from build123d import *

# Parameters (mm, degrees)
SKETCH1_W                                       = 295
SKETCH1_H                                       = 60
BOSS_EXTRUDE1_DEPTH                             = 3.175
FILLET1_R                                       = 10
F_3_0MM_DOWEL_HOLE1_D                           = 3
SKETCH6_R                                       = 12.5
CUT_EXTRUDE1_DEPTH                              = 242.888570679
F_6_0MM_DOWEL_HOLE1_D                           = 6
CSK_FOR_M3_FLAT_HEAD_MACHINE_SCREW1_D           = 3.4
CSK_FOR_M3_FLAT_HEAD_MACHINE_SCREW1_CSINK_D     = 6.3
CSK_FOR_M3_FLAT_HEAD_MACHINE_SCREW1_CSINK_ANGLE = 90
F_5_0MM_DOWEL_HOLE1_D                           = 5


with BuildPart() as part:
    # Sketch1 → Boss-Extrude1 (new body)
    with BuildSketch(Plane(origin=(0, 0, 0), x_dir=(1, 0, 0), z_dir=(0, 1, 0))):
        with Locations((92.5, 0)):
            Rectangle(SKETCH1_W, SKETCH1_H)
    extrude(amount=BOSS_EXTRUDE1_DEPTH)

    # Fillet1
    fillet1_edges = [part.edges().sort_by_distance(p)[0] for p in [
        (-55, 1.5875, -30),
        (240, 1.5875, -30),
        (240, 1.5875, 30),
        (-55, 1.5875, 30),
    ]]
    fillet(fillet1_edges, radius=FILLET1_R)

    # Ø3.0mm Dowel Hole1 (through all)
    with Locations(Plane(origin=(0, 3.175, 0), x_dir=(1, 0, 0), z_dir=(0, 1, 0))):
        with Locations((-15.5, 15.5), (15.5, 15.5), (15.5, -15.5), (-15.5, -15.5)):
            Hole(F_3_0MM_DOWEL_HOLE1_D / 2)

    # Sketch6 → Cut-Extrude1 (cut, through all)
    with BuildSketch(Plane(origin=(0, 3.175, 0), x_dir=(1, 0, 0), z_dir=(0, 1, 0))):
        with Locations(Location((0, 0, 0), (0, 0, 270))):
            Circle(SKETCH6_R)
    extrude(amount=-CUT_EXTRUDE1_DEPTH, mode=Mode.SUBTRACT)

    # Ø6.0mm Dowel Hole1 (through all)
    with Locations(Plane(origin=(0, 3.175, 0), x_dir=(1, 0, 0), z_dir=(0, 1, 0))):
        with Locations((200, 0)):
            Hole(F_6_0MM_DOWEL_HOLE1_D / 2)

    # CSK for M3 Flat Head Machine Screw1 (through all)
    with Locations(Plane(origin=(0, 0, 0), x_dir=(-1, 0, 0), z_dir=(0, -1, 0))):
        with Locations((-214, 9), (-186, 9), (-186, -9), (-214, -9)):
            CounterSinkHole(CSK_FOR_M3_FLAT_HEAD_MACHINE_SCREW1_D / 2, CSK_FOR_M3_FLAT_HEAD_MACHINE_SCREW1_CSINK_D / 2, counter_sink_angle=CSK_FOR_M3_FLAT_HEAD_MACHINE_SCREW1_CSINK_ANGLE)

    # Ø5.0mm Dowel Hole1 (through all)
    with Locations(Plane(origin=(0, 3.175, 0), x_dir=(1, 0, 0), z_dir=(0, 1, 0))):
        with Locations((55, -25), (110, -25), (165, -25), (165, 25), (110, 25), (55, 25), (-40, -25), (-40, 25)):
            Hole(F_5_0MM_DOWEL_HOLE1_D / 2)


solid = part.part
Can you work these out from the model? Positions are in its coordinate system, mm. Coordinates: 2 decimals unless noted, no trailing zeros. Write each loop counter-clockwise with the first axis right and the second up, starting at its lowest first coordinate (ties: lowest second). Pieces come first, ordered by that corner, then holes. Notation, with made-up numbers: (40, 83.5) -> (95, 83.5) arc R26 ccw to (95, 119.5) -> close; hole circle Ø1 at (44.5, 20.25). An arc over 180 degrees is marked (long way). Write item = value, one per line.
(1) Imagine slicing it at D-D (y = 0.55). State how many separate pieces and enclosed holes the cut face has, and give its area (3 significant figures).
Verdict:
separate_pieces = 1
enclosed_holes = 18
area = 16,800 mm^2
(2) Imagine slicing it at B-B (x = 110). Please give me the cut outline in (y, z) (3 decimals), and give its area (3 significant figures).
Verdict:
outline = (0, -30) -> (3.175, -30) -> (3.175, -27.5) -> (0, -27.5) -> close; (0, -22.5) -> (3.175, -22.5) -> (3.175, 22.5) -> (0, 22.5) -> close; (0, 27.5) -> (3.175, 27.5) -> (3.175, 30) -> (0, 30) -> close
area = 159 mm^2
(3) Imagine slicing it at C-C (z = 0). Please give me the cut outline in (x, y) (3 decimals), and give its area (3 significant figures).
Verdict:
outline = (-55, 0) -> (-12.5, 0) -> (-12.5, 3.175) -> (-55, 3.175) -> close; (12.5, 0) -> (197, 0) -> (197, 3.175) -> (12.5, 3.175) -> close; (203, 0) -> (240, 0) -> (240, 3.175) -> (203, 3.175) -> close
area = 838 mm^2
(4) Imagine slicing it at A-A (x = 200). Please give me the cut outline in (y, z) (3 decimals), and give its area (3 significant figures).
Verdict:
outline = (0, -30) -> (3.175, -30) -> (3.175, -3) -> (0, -3) -> close; (0, 3) -> (3.175, 3) -> (3.175, 30) -> (0, 30) -> close
area = 171 mm^2
(5) If I drill on probe 1 along Z at (x, y) = (15.5, 2.2); probe 2 along Z at (x, y) = (55, 0.8); probe 3 along X at (y, z) = (2, -0.5), over which ranges is the centre line in solid material (lowest first)?
Verdict:
probe_1 = -30 to -17, -14 to 14, 17 to 30
probe_2 = -30 to -27.5, -22.5 to 22.5, 27.5 to 30
probe_3 = -55 to -12.49, 12.49 to 197.04, 202.96 to 240
(6) Thinking about a two-plate mould opening in Z: for faces 1 (the face through (237.15, 1.61, -26.99)), 2 (the face through (-41.34, 1.57, -27.11)), 3 (the face through (3.755, 1.61, 11.923)), 4 (the face through (-52.15, 1.61, 26.99)), which applies, +Z half, -Z half, draft (parallel to the pull), parting line (faces both ways), or undercut?
Verdict:
face_1 = -Z half
face_2 = undercut
face_3 = undercut
face_4 = +Z half
